Source: CAD feature listing. Evaluate the final solid. Frame: model axes, mm. Round coordinates to 2 decimals unless told otherwise and drop trailing zeros. Write each loop counter-clockwise with the first axis right and the second up, starting at its lowest first coordinate (ties: lowest second). Pieces come first, ordered by that corner, then holes. Notation, with made-up numbers: M -3.75,23.5 L 17.25,23.5 A18 cw 17.25,56.5 Z; hole C -24,89 d5. An arc over 180 degrees is marked long. Answer in a Markdown table with one row per item.
from build123d import *

# Parameters (mm, degrees)
SKETCH1_W               = 717
SKETCH1_H               = 25
SKETCH1_R               = 7.5
BOSS_EXTRUDE1_DEPTH     = 25
FILLET1_R               = 12
CUT_EXTRUDE1_DEPTH      = 718.544597917
CUT_EXTRUDE1_DEPTH_BACK = 718.544597917
SKETCH2_W               = 12.5
SKETCH2_H               = 25


with BuildPart() as part:
    # Sketch1 → Boss-Extrude1 (new body)
    with BuildSketch(Plane.XY):
        Rectangle(SKETCH1_W, SKETCH1_H)
        with Locations((-338.5, 0)):
            Circle(SKETCH1_R, mode=Mode.SUBTRACT)
        with Locations((338.5, 0)):
            Circle(SKETCH1_R, mode=Mode.SUBTRACT)
    extrude(amount=BOSS_EXTRUDE1_DEPTH)

    # Fillet1
    fillet1_edges = [part.edges().sort_by_distance(p)[0] for p in [
        (-358.5, -12.5, 12.5),
        (-358.5, 12.5, 12.5),
    ]]
    fillet(fillet1_edges, radius=FILLET1_R)

    # Sketch2 → Cut-Extrude1 (cut, two sides: drawn at the far end of the back side and taken through both)
    with BuildSketch(Plane(origin=(358.5, 0, 0), x_dir=(0, 0, -1), z_dir=(1, 0, 0)).offset(-CUT_EXTRUDE1_DEPTH_BACK)):
        with Locations((-6.25, 0)):
            Rectangle(SKETCH2_W, SKETCH2_H)
    extrude(amount=CUT_EXTRUDE1_DEPTH + CUT_EXTRUDE1_DEPTH_BACK, mode=Mode.SUBTRACT)


solid = part.part
Q1. Section B-B (z = 21). Return loops of the section in (x, y), and give its area (3 significant figures).
Solutions:
| item | result |
|---|---|
| outline | M -358.5,-0.5 A12 ccw -346.5,-12.5 L 358.5,-12.5 L 358.5,12.5 L -346.5,12.5 A12 ccw -358.5,0.5 Z; hole C -338.5,0 d15; hole C 338.5,0 d15 |
| area | 17,500 mm2 |
Q2. Contact query for a flat-ended pin moving along its axis: pin 1 Ø2 at (y, z) = (-5, 21) entering from -X. Output: stop coordinate, or through.
Solutions:
| item | result |
|---|---|
| pin 1 | stops at x = -357.98 |
Q3. Section A-A (x = 338.5). Return loops of the section in (y, z).
Solutions:
| item | result |
|---|---|
| outline | M -12.5,12.5 L -7.5,12.5 L -7.5,25 L -12.5,25 Z; M 7.5,12.5 L 12.5,12.5 L 12.5,25 L 7.5,25 Z |
Q4. Material intervals for probe 1 along X at (y, z) = (0, 18.5); probe 2 along Y at (x, z) = (-338.5, 16); probe 3 along X at (y, z) = (5.5, 16.5), sorted ascending.
Solutions:
| item | result |
|---|---|
| probe 1 | x = -358.5 to -346, -331 to 331, 346 to 358.5 |
| probe 2 | y = -12.5 to -7.5, 7.5 to 12.5 |
| probe 3 | x = -357.41 to -343.6, -333.4 to 333.4, 343.6 to 358.5 |
